Source: CAD feature listing. Evaluate the final solid. Frame: model axes, mm. Face numbers are marked on the shaded views. A direction names the side the tool comes from. Give positions to 0.01 mm unless a question says otherwise; leave off trailing zeros. Loops run counter-clockwise (first coordinate to the right, second up) from the corner with the lowest first, then second, coordinate; pieces in that order, holes last. Notation, with made-up numbers: (6, -20.5) -> (12, -20.5) arc R8 cw to (12, -11.5) -> close; hole circle Ø8 at (20, 86.25). An arc over 180 degrees is marked (long way). Answer as a JSON object with one key per item and string values. Group by question number.
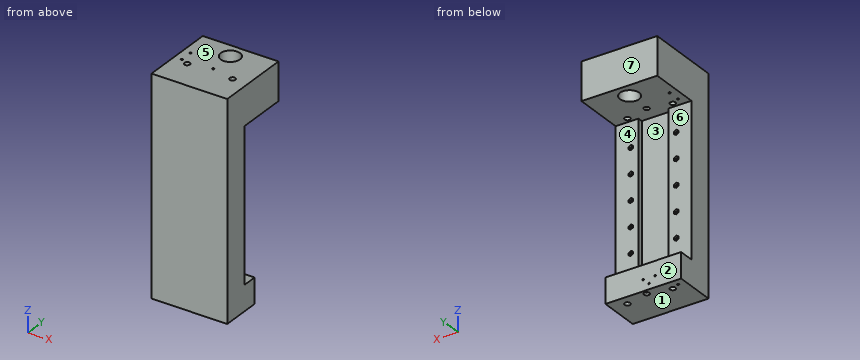
from build123d import *

# Parameters (mm, degrees)
RESSALTO_EXTRUS_O1_DEPTH                        = 150
CORTE_EXTRUS_O1_REACH                           = 915.783
ESBO_O2_R                                       = 38.1
ESBO_O2_R_2                                     = 4
ESBO_O2_R_3                                     = 11.11
SKETCH2_W                                       = 120
SKETCH2_H                                       = 600
CUT_EXTRUDE2_DEPTH                              = 20
CSK_FOR_M3_FLAT_HEAD_MACHINE_SCREW1_D           = 3.4
CSK_FOR_M3_FLAT_HEAD_MACHINE_SCREW1_DEPTH       = 10
CSK_FOR_M3_FLAT_HEAD_MACHINE_SCREW1_CSINK_D     = 6.3
CSK_FOR_M3_FLAT_HEAD_MACHINE_SCREW1_CSINK_ANGLE = 90
CSK_FOR_M3_FLAT_HEAD_MACHINE_SCREW1_TIP         = 1.021463052
SKETCH6_R                                       = 11
CUT_EXTRUDE3_DEPTH                              = 10
LPATTERN1_COUNT                                 = 2
LPATTERN1_PITCH                                 = 90
CUT_EXTRUDE4_START                              = 610
SKETCH6_2_R                                     = 11
CUT_EXTRUDE4_DEPTH                              = 10
TAP_DRILL_FOR_M10X1_0_TAP1_D                    = 9
TAP_DRILL_FOR_M10X1_0_TAP1_DEPTH                = 20
TAP_DRILL_FOR_M10X1_0_TAP1_TIP                  = 2.703872786
CUT_EXTRUDE5_DEPTH                              = 8


with BuildPart() as part:
    # Esboço1 → Ressalto-extrusão1 (new, symmetric)
    with BuildSketch(Plane(origin=(0, 0, 0), x_dir=(0, 0, -1), z_dir=(1, 0, 0))):
        Polygon((0, 0), (850, 0), (850, 160), (750, 160), (750, 100), (150, 100), (150, 300), (0, 300), align=None)
    extrude(amount=RESSALTO_EXTRUS_O1_DEPTH, both=True)

    # Corte-extrusão1: up to this face of the body (flat: up to its plane)
    corte_extrus_o1_end = Plane(part.part.faces().sort_by_distance((0, 80, -850))[0])
    # Esboço2 → Corte-extrusão1 (cut, up to the picked face)
    with BuildSketch(Plane.XY, mode=Mode.PRIVATE) as corte_extrus_o1_sk1:
        with Locations((0, 240)):
            Circle(ESBO_O2_R)
    corte_extrus_o1_tool1 = split(extrude(corte_extrus_o1_sk1.sketch, amount=-CORTE_EXTRUS_O1_REACH, mode=Mode.PRIVATE), bisect_by=corte_extrus_o1_end, keep=Keep.BOTH, mode=Mode.PRIVATE)
    # Esboço2 → Corte-extrusão1 (cut, up to the picked face)
    with BuildSketch(Plane.XY, mode=Mode.PRIVATE) as corte_extrus_o1_sk2:
        with Locations((0, 140)):
            Circle(ESBO_O2_R_2)
    corte_extrus_o1_tool2 = split(extrude(corte_extrus_o1_sk2.sketch, amount=-CORTE_EXTRUS_O1_REACH, mode=Mode.PRIVATE), bisect_by=corte_extrus_o1_end, keep=Keep.BOTH, mode=Mode.PRIVATE)
    # Esboço2 → Corte-extrusão1 (cut, up to the picked face)
    with BuildSketch(Plane.XY, mode=Mode.PRIVATE) as corte_extrus_o1_sk3:
        with Locations((-90, 120)):
            Circle(ESBO_O2_R_3)
    corte_extrus_o1_tool3 = split(extrude(corte_extrus_o1_sk3.sketch, amount=-CORTE_EXTRUS_O1_REACH, mode=Mode.PRIVATE), bisect_by=corte_extrus_o1_end, keep=Keep.BOTH, mode=Mode.PRIVATE)
    # Esboço2 → Corte-extrusão1 (cut, up to the picked face)
    with BuildSketch(Plane.XY, mode=Mode.PRIVATE) as corte_extrus_o1_sk4:
        with Locations((90, 120)):
            Circle(ESBO_O2_R_3)
    corte_extrus_o1_tool4 = split(extrude(corte_extrus_o1_sk4.sketch, amount=-CORTE_EXTRUS_O1_REACH, mode=Mode.PRIVATE), bisect_by=corte_extrus_o1_end, keep=Keep.BOTH, mode=Mode.PRIVATE)
    # Esboço2 → Corte-extrusão1 (cut, up to the picked face)
    with BuildSketch(Plane.XY, mode=Mode.PRIVATE) as corte_extrus_o1_sk5:
        with Locations((-120, 183.762072292)):
            Circle(ESBO_O2_R_2)
    corte_extrus_o1_tool5 = split(extrude(corte_extrus_o1_sk5.sketch, amount=-CORTE_EXTRUS_O1_REACH, mode=Mode.PRIVATE), bisect_by=corte_extrus_o1_end, keep=Keep.BOTH, mode=Mode.PRIVATE)
    # Esboço2 → Corte-extrusão1 (cut, up to the picked face)
    with BuildSketch(Plane.XY, mode=Mode.PRIVATE) as corte_extrus_o1_sk6:
        with Locations((-120, 133.762072292)):
            Circle(ESBO_O2_R_2)
    corte_extrus_o1_tool6 = split(extrude(corte_extrus_o1_sk6.sketch, amount=-CORTE_EXTRUS_O1_REACH, mode=Mode.PRIVATE), bisect_by=corte_extrus_o1_end, keep=Keep.BOTH, mode=Mode.PRIVATE)
    add(corte_extrus_o1_tool1.solids().sort_by(Axis((0, 240, 0), (0, 0, -1)))[0], mode=Mode.SUBTRACT)
    add(corte_extrus_o1_tool2.solids().sort_by(Axis((0, 140, 0), (0, 0, -1)))[0], mode=Mode.SUBTRACT)
    add(corte_extrus_o1_tool3.solids().sort_by(Axis((-90, 120, 0), (0, 0, -1)))[0], mode=Mode.SUBTRACT)
    add(corte_extrus_o1_tool4.solids().sort_by(Axis((90, 120, 0), (0, 0, -1)))[0], mode=Mode.SUBTRACT)
    add(corte_extrus_o1_tool5.solids().sort_by(Axis((-120, 183.762072, 0), (0, 0, -1)))[0], mode=Mode.SUBTRACT)
    add(corte_extrus_o1_tool6.solids().sort_by(Axis((-120, 133.762072, 0), (0, 0, -1)))[0], mode=Mode.SUBTRACT)

    # Sketch2 → Cut-Extrude2 (cut)
    with BuildSketch(Plane(origin=(0, 100, 0), x_dir=(1, 0, 0), z_dir=(0, 1, 0))):
        with Locations((0, 450)):
            Rectangle(SKETCH2_W, SKETCH2_H)
    extrude(amount=-CUT_EXTRUDE2_DEPTH, mode=Mode.SUBTRACT)

    # CSK for M3 Flat Head Machine Screw1
    with Locations(Plane(origin=(0, 160, 0), x_dir=(1, 0, 0), z_dir=(0, 1, 0))):
        with Locations((-46.6, 806), (-23.05, 828), (0.5, 806)):
            CounterSinkHole(CSK_FOR_M3_FLAT_HEAD_MACHINE_SCREW1_D / 2, CSK_FOR_M3_FLAT_HEAD_MACHINE_SCREW1_CSINK_D / 2, depth=CSK_FOR_M3_FLAT_HEAD_MACHINE_SCREW1_DEPTH, counter_sink_angle=CSK_FOR_M3_FLAT_HEAD_MACHINE_SCREW1_CSINK_ANGLE)
            with Locations((0, 0, -(CSK_FOR_M3_FLAT_HEAD_MACHINE_SCREW1_DEPTH + CSK_FOR_M3_FLAT_HEAD_MACHINE_SCREW1_TIP / 2))):  # 118° drill point
                Cone(0, CSK_FOR_M3_FLAT_HEAD_MACHINE_SCREW1_D / 2, CSK_FOR_M3_FLAT_HEAD_MACHINE_SCREW1_TIP, mode=Mode.SUBTRACT)

    # Sketch6 → Cut-Extrude3 (cut)
    with BuildSketch(Plane.XY.offset(-750)):
        with Locations((0, 140)):
            Circle(SKETCH6_R)
    cut_extrude3 = extrude(amount=-CUT_EXTRUDE3_DEPTH, mode=Mode.SUBTRACT)

    # LPattern1: Cut-Extrude3 ×2
    with Locations(*[(0, 0, -i * LPATTERN1_PITCH) for i in range(1, LPATTERN1_COUNT)]):
        add(cut_extrude3, mode=Mode.SUBTRACT)

    # Sketch6<2> → Cut-Extrude4 (cut)
    with BuildSketch(Plane.XY.offset(-750).offset(CUT_EXTRUDE4_START)):
        with Locations((0, 140)):
            Circle(SKETCH6_2_R)
    extrude(amount=-CUT_EXTRUDE4_DEPTH, mode=Mode.SUBTRACT)

    # Tap Drill for M10x1.0 Tap1
    with Locations(Plane(origin=(0, 100, 0), x_dir=(1, 0, 0), z_dir=(0, 1, 0))):
        with Locations((-90, 650), (90, 650), (-90, 550), (90, 550), (90, 450), (-90, 450), (-90, 350), (-90, 250), (90, 250), (90, 350)):
            Hole(TAP_DRILL_FOR_M10X1_0_TAP1_D / 2, depth=TAP_DRILL_FOR_M10X1_0_TAP1_DEPTH)
            with Locations((0, 0, -(TAP_DRILL_FOR_M10X1_0_TAP1_DEPTH + TAP_DRILL_FOR_M10X1_0_TAP1_TIP / 2))):  # 118° drill point
                Cone(0, TAP_DRILL_FOR_M10X1_0_TAP1_D / 2, TAP_DRILL_FOR_M10X1_0_TAP1_TIP, mode=Mode.SUBTRACT)

    # Sketch10 → Cut-Extrude5 (cut)
    with BuildSketch(Plane(origin=(0, 100, 0), x_dir=(1, 0, 0), z_dir=(0, 1, 0))):
        Polygon((-98.5, 645.092522712), (-90, 640.185045424), (-81.5, 645.092522712), (-81.5, 654.907477288), (-90, 659.814954576), (-98.5, 654.907477288), align=None)
        Polygon((98.5, 654.907477288), (98.5, 645.092522712), (90, 640.185045424), (81.5, 645.092522712), (81.5, 654.907477288), (90, 659.814954576), align=None)
        Polygon((-98.5, 545.092522712), (-90, 540.185045424), (-81.5, 545.092522712), (-81.5, 554.907477288), (-90, 559.814954576), (-98.5, 554.907477288), align=None)
        Polygon((98.5, 554.907477288), (98.5, 545.092522712), (90, 540.185045424), (81.5, 545.092522712), (81.5, 554.907477288), (90, 559.814954576), align=None)
        Polygon((-98.5, 445.092522712), (-90, 440.185045424), (-81.5, 445.092522712), (-81.5, 454.907477288), (-90, 459.814954576), (-98.5, 454.907477288), align=None)
        Polygon((98.5, 454.907477288), (98.5, 445.092522712), (90, 440.185045424), (81.5, 445.092522712), (81.5, 454.907477288), (90, 459.814954576), align=None)
        Polygon((-98.5, 345.092522712), (-90, 340.185045424), (-81.5, 345.092522712), (-81.5, 354.907477288), (-90, 359.814954576), (-98.5, 354.907477288), align=None)
        Polygon((98.5, 354.907477288), (98.5, 345.092522712), (90, 340.185045424), (81.5, 345.092522712), (81.5, 354.907477288), (90, 359.814954576), align=None)
        Polygon((-98.5, 245.092522712), (-90, 240.185045424), (-81.5, 245.092522712), (-81.5, 254.907477288), (-90, 259.814954576), (-98.5, 254.907477288), align=None)
        Polygon((98.5, 254.907477288), (98.5, 245.092522712), (90, 240.185045424), (81.5, 245.092522712), (81.5, 254.907477288), (90, 259.814954576), align=None)
    extrude(amount=-CUT_EXTRUDE5_DEPTH, mode=Mode.SUBTRACT)


solid = part.part
(1) Section query C-C on z = -99.5. Return the cut outline in (x, y).
(2) Section query A-A on z = -741. Return the cut outline in (x, y).
(3) Material intervals for line 1 (Z direction, x = -90, y = 87.25); line 2 (X direction, y = 84.5, z = -650); line 3 (Y direction, x = 0, z = -37.5), sorted ascending. Write a range as from..to.
(4) Access query for the marked faces 1, 2, 3 and 4. Directions: +Z, -Z, +X, -X, +Y, -Y. A direction counts if a zero-diameter tool reaches every point of the face in a straight line with its end or side. Return the directions, or none.
(5) Section query B-B on y = 210.5. Return the cut outline in (x, z).
(6) First-contact query: pin 1 (12 mm diameter, centred on x = 7, z = -338.5, fed in from +Y); pin 2 (8.5 mm diameter, centred on x = -86, z = -453, fed in from +Y); pin 3 (11.5 mm diameter, centred on x = -90, z = -350, fed in from +Y). Flat tips, straight axial feed; report the tip coordinate or a pass-through.
(7) Mould query, pull axis Z, two halves, no side actions, for the marked faces 5, 6 and 7. Classes: pulls with the +Z half, pulls with the -Z half, needs draft (parallel to the pull), parting line crosses it, or undercut.
Result:
{
 "1": {"outline": "(-150, 0) -> (150, 0) -> (150, 300) -> (-150, 300) -> close; hole circle Ø8 at (-120, 133.76); hole circle Ø8 at (-120, 183.76); hole circle Ø22.22 at (-90, 120); hole circle Ø76.2 at (0, 240); hole circle Ø8 at (0, 140); hole circle Ø22.22 at (90, 120)"},
 "2": {"outline": "(-150, 0) -> (150, 0) -> (150, 100) -> (60, 100) -> (60, 80) -> (-60, 80) -> (-60, 100) -> (-150, 100) -> close"},
 "3": {"line 1": "-850..-654.5, -645.5..-554.5, -545.5..-454.5, -445.5..-354.5, -345.5..-254.5, -245.5..0", "line 2": "-150..-94.5, -85.5..-60, 60..85.5, 94.5..150", "line 3": "0..136, 144..201.9, 278.1..300"},
 "4": {"face 1": "-Z, +X, -X, +Y, -Y", "face 2": "-Z, +X, -X, +Y", "face 3": "+Y", "face 4": "+X, -X, +Y"},
 "5": {"outline": "(-150, -150) -> (-24.11, -150) -> (-24.11, 0) -> (-150, 0) -> close; (24.11, -150) -> (150, -150) -> (150, 0) -> (24.11, 0) -> close"},
 "6": {"pin 1": "y = 80", "pin 2": "y = 100", "pin 3": "y = 92"},
 "7": {"face 5": "pulls with the +Z half", "face 6": "undercut", "face 7": "needs draft"}
}
